```python
from build123d import *

# Parameters (mm, degrees)
F1_DEPTH = 400
F2_R     = 150
F3_DEPTH = 100
F4_W     = 900
F4_H     = 300
F5_DEPTH = 400


with BuildPart() as f1:
    # F0 (on Front) → F1 (new body)
    with BuildSketch(Plane.XZ):
        Polygon((-931.680651, 397.194484), (-1031.680651, 397.194484), (-1031.680651, -2.805516), (-1031.680651, -47.295272), (-31.680651, -47.295272), (-31.680651, 52.704728), (-31.680651, 397.194484), (-131.680651, 397.194484), (-431.680651, 397.194484), (-631.680651, 397.194484), align=None)
    extrude(amount=-F1_DEPTH)

    # F2 (on face) → F3 (join)
    with BuildSketch(Plane.XY.offset(397.194484)):
        with Locations((-781.680651, 200)):
            Circle(F2_R)
        with Locations((-281.680651, 200)):
            Circle(F2_R)
    extrude(amount=F3_DEPTH)

    # F4 (on face) → F5 (cut)
    with BuildSketch(Plane(origin=(0, 0, -47.295272), x_dir=(1, 0, 0), z_dir=(0, 0, -1))):
        with Locations((-531.680651, -200)):
            Rectangle(F4_W, F4_H)
    extrude(amount=-F5_DEPTH, mode=Mode.SUBTRACT)


solid = f1.part
```
Source: CAD feature listing. Evaluate the final solid. Frame: model axes, mm. A direction names the side the tool comes from. Round coordinates to 2 decimals unless told otherwise and drop trailing zeros. Loops run counter-clockwise (first coordinate to the right, second up) from the corner with the lowest first, then second, coordinate; pieces in that order, holes last.
1. Section query B-B on x = -591. Output: boundary loops of the cut face in (y, z).
2. Section query A-A on z = 11. Output: boundary loops of the cut face in (x, y), and give its area (3 significant figures).
3. Ray query, L1, parallel to X at y = 157, z = 170.5; L2, parallel to Y at x = -624.5, z = 83.5; L3, parallel to Z at x = -849, y = 285. Return the intervals inside material, ascending.
4. Section query C-C on y = 200. Output: boundary loops of the cut face in (x, z), and give its area (3 significant figures).
5. Contact query for a flat-ended pin moving along its axis: pin 1 (1.5 mm diameter, centred on x = -160.5, y = 47.5, fed in from +Z). Output: stop coordinate, or through.
6. Mould query, pull axis Y, two halves, no side actions, for faces 4 (the flat face through (-784, 202, 497.194)), 5 (the flat face through (-538, 350, 150)), 6 (the cylindrical face through (-643.12, 142.55, 446.49)). Classes: released by +Y, released by -Y, zero draft, split by the parting line, or undercut.
7. Access query for faces 1 (the flat face through (-539, 0, 178)), 2 (the cylindrical face through (-314.198, 53.567, 446.494)), 3 (the flat face through (-538, 50, 150)). Directions: +Z, -Z, +X, -X, +Y, -Y. A direction counts if a zero-diameter tool reaches every point of the face in a straight line with its end or side. Return the directions, or none.
8. Section query D-D on y = 251. Output: boundary loops of the cut face in (x, z).
Answers below:
1. outline: (0, -47.3) - (50, -47.3) - (50, 352.7) - (350, 352.7) - (350, -47.3) - (400, -47.3) - (400, 397.19) - (0, 397.19) - close
2. outline: (-1031.68, 0) - (-31.68, 0) - (-31.68, 400) - (-1031.68, 400) - close; hole (-981.68, 50) - (-81.68, 50) - (-81.68, 350) - (-981.68, 350) - close
2. area: 130,000 mm2
3. L1: x = -1031.68 to -981.68, -81.68 to -31.68
3. L2: y = 0 to 50, 350 to 400
3. L3: z = 352.7 to 497.19
4. outline: (-1031.68, -47.3) - (-981.68, -47.3) - (-981.68, 352.7) - (-81.68, 352.7) - (-81.68, -47.3) - (-31.68, -47.3) - (-31.68, 397.19) - (-131.68, 397.19) - (-131.68, 497.19) - (-431.68, 497.19) - (-431.68, 397.19) - (-631.68, 397.19) - (-631.68, 497.19) - (-931.68, 497.19) - (-931.68, 397.19) - (-1031.68, 397.19) - close
4. area: 144,000 mm2
5. pin 1: stops at z = 397.19
6. face 4: zero draft
6. face 5: undercut
6. face 6: split by the parting line
7. face 1: +Z, -Z, +X, -X, -Y
7. face 2: +Z
7. face 3: -Z
8. outline: (-1031.68, -47.3) - (-981.68, -47.3) - (-981.68, 352.7) - (-81.68, 352.7) - (-81.68, -47.3) - (-31.68, -47.3) - (-31.68, 397.19) - (-140.62, 397.19) - (-140.62, 497.19) - (-422.74, 497.19) - (-422.74, 397.19) - (-640.62, 397.19) - (-640.62, 497.19) - (-922.74, 497.19) - (-922.74, 397.19) - (-1031.68, 397.19) - close
